Autodesk Inventor part; units mm, degrees
ref_plane "YZ Plane" through (0, 0, 0) normal (1, 0, 0) x (0, 1, 0)
ref_plane "XZ Plane" through (0, 0, 0) normal (0, 1, 0) x (-1, 0, 0)
ref_plane "XY Plane" through (0, 0, 0) normal (0, 0, 1) x (1, 0, 0)
sketch "スケッチ1" plane through (0, 0, 0) normal (0, 0, 1) x (1, 0, 0)
  line L0 (10, -2.5) -> (-10, -2.5)
  line L1 (-10, -2.5) -> (-10, 2.5)
  line L2 (-10, 2.5) -> (10, 2.5)
  line L3 (10, 2.5) -> (10, -2.5)
  line L4 (10, -2.5) -> (-10, 2.5) construction
  line L5 (-10, -2.5) -> (10, 2.5) construction
  circle A0 centre (-7.5, 0) radius 1.1
  circle A1 centre (7.5, 0) radius 1.1
  line L6 (5.5, -2.5) -> (5.5, 2.5)
  line L7 (-5.5, 2.5) -> (-5.5, -2.5)
  line L8 (-5.5, -1.5) -> (5.5, -1.5)
  line L9 (-5.5, 1.5) -> (5.5, 1.5)
  line L10 (3, -1.5) -> (3, 1.5)
  line L11 (3, 1.5) -> (3.4, 1.5)
  line L12 (3.4, 1.5) -> (3.4, -1.5)
  line L13 (3, -1.5) -> (2.6, -1.5)
  line L14 (2.6, -1.5) -> (2.6, 1.5)
  line L15 (-3, -1.5) -> (-3, 1.5)
  line L16 (-3, 1.5) -> (-3.4, 1.5)
  line L17 (-3.4, 1.5) -> (-3.4, -1.5)
  line L18 (-3, -1.5) -> (-2.6, -1.5)
  line L19 (-2.6, -1.5) -> (-2.6, 1.5)
  point P0 (0, 0)
  dimension "d0" = 20
  dimension "d1" = 5
  dimension "d2" = 2.2
  dimension "d3" = 2.2
  dimension "d4" = 0.4
  dimension "d5" = 0.4
  dimension "d6" = 0.4
  dimension "d7" = 0.4
  dimension "d10" = 1
  dimension "d11" = 1
  dimension "d16" = 2.5
  dimension "d17" = 4.5
  dimension "d18" = 2.1
extrude "押し出し1" add sketch "スケッチ1" along normal blind 8 contours L0 L6 L2 L3 | L0 L7 L8 L6 | L0 L1 L2 L7 | L6 L9 L7 L2 | L8 L10 L9 L12 | L17 L9 L15 L8 | L8 L14 L9 L10 | L15 L9 L19 L8
sketch "スケッチ2" plane through (0, 0, 8) normal (0, 0, 1) x (1, 0, 0)
  circle A0 centre (-7.5, 0) radius 1.1
  circle A1 centre (-7.5, 0) radius 1.85
  circle A2 centre (7.5, 0) radius 1.1
  circle A3 centre (7.5, 0) radius 1.85
  point P0 (0, 0)
  dimension "d12" = 3.7
  dimension "d13" = 3.7
extrude "押し出し2" cut sketch "スケッチ2" against normal blind 2 contours A0 | A1 | A3
properties part number "griper_TPU" material "ゴム、シリコーン"
Input: part model. Units: mm. Frame: model coordinates. A direction names the side the tool comes from. Round coordinates to 2 decimals unless told otherwise and drop trailing zeros. Loops run counter-clockwise (first coordinate to the right, second up) from the corner with the lowest first, then second, coordinate; pieces in that order, holes last. Notation, with made-up numbers: M 54.25,89 L 61.25,89 A14 ccw 61.25,107 Z; hole C 77,11.25 d3. An arc over 180 degrees is marked long. Answer in a Markdown table with one row per item. Add a question column.
1. Section D-D (x = 0.25). Output: boundary loops of the cut face in (y, z).
2. Section B-B (z = 2.5). Output: boundary loops of the cut face in (x, y).
3. Mould query, pull axis X, two halves, no side actions, for faces 4 (the face through (3.4, 0, 4)), 5 (the face through (10, 0, 4)), 6 (the face through (0, 2, 8)). Classes: released by +X, released by -X, zero draft, split by the parting line, or undercut.
4. Contact query for flat-ended pins moving along their axis: pin 1 (1.1 mm diameter, centred on x = -7, y = 0, fed in from +Z) (3 decimals); pin 2 (3 mm diameter, centred on x = 7.5, y = 0, fed in from +Z). Output: stop coordinate, or through.
5. Set-up query: faces 1 (the face through (-6, 0, 6)), 2 (the face through (-5.5, 0, 4)), 3 (the face through (0, 2, 0)). Return all of +Z, -Z, +X, -X, +Y, -Y with unobstructed straight access to the full face (end or side cutting, diameter ignored); none if empty.
6. Ray query, probe 1 along X at (y, z) = (-1.25, 5.75); probe 2 along Y at (x, z) = (-3.75, 6.25); probe 3 along Y at (x, z) = (7.5, 3). Return the intervals inside material, ascending.
7. Section C-C (y = 0.9). Give the number of separate pieces and of enclosed holes in the cut face, and give its area (3 significant figures).
8. Section A-A (x = -7.5). Output: boundary loops of the cut face in (y, z).
Values follow:
| question | item | result |
|---|---|---|
| 1 | outline | M -2.5,0 L -1.5,0 L -1.5,8 L -2.5,8 Z; M 1.5,0 L 2.5,0 L 2.5,8 L 1.5,8 Z |
| 2 | outline | M -10,-2.5 L 10,-2.5 L 10,2.5 L -10,2.5 Z; hole C -7.5,0 d2.2; hole M -5.5,-1.5 L -3.4,-1.5 L -3.4,1.5 L -5.5,1.5 Z; hole M -2.6,-1.5 L 2.6,-1.5 L 2.6,1.5 L -2.6,1.5 Z; hole M 3.4,-1.5 L 5.5,-1.5 L 5.5,1.5 L 3.4,1.5 Z; hole C 7.5,0 d2.2 |
| 3 | face 4 | undercut |
| 3 | face 5 | released by +X |
| 3 | face 6 | zero draft |
| 4 | pin 1 | through |
| 4 | pin 2 | z = 6 |
| 5 | face 1 | +Z |
| 5 | face 2 | +Z, -Z |
| 5 | face 3 | -Z, +X, -X, +Y, -Y |
| 6 | probe 1 | -10 to -5.5, -3.4 to -2.6, 2.6 to 3.4, 5.5 to 10 |
| 6 | probe 2 | -2.5 to -1.5, 1.5 to 2.5 |
| 6 | probe 3 | -2.5 to -1.1, 1.1 to 2.5 |
| 7 | separate pieces | 6 |
| 7 | enclosed holes | 0 |
| 7 | area | 56.7 mm^2 |
| 8 | outline | M -2.5,0 L -1.1,0 L -1.1,6 L -1.85,6 L -1.85,8 L -2.5,8 Z; M 1.1,0 L 2.5,0 L 2.5,8 L 1.85,8 L 1.85,6 L 1.1,6 Z |
